```python
from build123d import *

# Parameters (mm, degrees)
SKETCH_W     = 65
SKETCH_H     = 56
SKETCH_R     = 1.5
PAD_DEPTH    = 1
FILLET_R     = 5
SKETCH001_W  = 40
SKETCH001_H  = 5
PAD001_DEPTH = 18
SKETCH002_W  = 5
SKETCH002_H  = 35
PAD002_DEPTH = 12


with BuildPart() as part:
    # Sketch → Pad (new body)
    with BuildSketch(Plane.XY):
        Rectangle(SKETCH_W, SKETCH_H)
        with Locations((-26.696429, 23)):
            Circle(SKETCH_R, mode=Mode.SUBTRACT)
        with Locations((-26.696429, -23)):
            Circle(SKETCH_R, mode=Mode.SUBTRACT)
        with Locations((26.696429, -23)):
            Circle(SKETCH_R, mode=Mode.SUBTRACT)
        with Locations((26.696429, 23)):
            Circle(SKETCH_R, mode=Mode.SUBTRACT)
    extrude(amount=PAD_DEPTH)

    # Fillet
    fillet_edges = [part.edges().sort_by_distance(p)[0] for p in [
        (-32.5, -28, 0.5),
        (32.5, -28, 0.5),
        (32.5, 28, 0.5),
        (-32.5, 28, 0.5),
    ]]
    fillet(fillet_edges, radius=FILLET_R)

    # Sketch001 (on Face5 of Fillet) → Pad001 (join)
    with BuildSketch(Plane.XY.offset(1)):
        with Locations((0, -23)):
            Rectangle(SKETCH001_W, SKETCH001_H)
    extrude(amount=PAD001_DEPTH)

    # Sketch002 (on Face2 of Pad001) → Pad002 (join)
    with BuildSketch(Plane(origin=(0, 0, 0), x_dir=(1, 0, 0), z_dir=(0, 0, -1))):
        with Locations((20, 0)):
            Rectangle(SKETCH002_W, SKETCH002_H)
    extrude(amount=PAD002_DEPTH)


solid = part.part
```
Geometry: final body of the model. Coordinates: model frame, mm. A direction names the side the tool comes from. Coordinates: 2 decimals unless noted, no trailing zeros. Order: outer loops, then holes, each group sorted by start corner. A loop starts at its lowest first (then second) coordinate and runs counter-clockwise, first axis right, second up. Notation, with made-up numbers: (68, 77.25) -> (109, 77.25) arc R24 cw to (109, 98.25) -> close; hole circle Ø2 at (38.5, -33). An arc over 180 degrees is marked (long way). Write each question's results on one line, items separated by ' | '. Start each with the question number.
1) Cut plane A-A, the plane y = -11.5. Output: boundary loops of the cut face in (x, z), and give its area (3 significant figures).
2) Mould query, pull axis X, two halves, no side actions, for faces 1 (the flat face through (-20, -23, 10)), 2 (the flat face through (0, -25.5, 10)), 3 (the cylindrical face through (27.503, 24.265, 0.493)). Classes: released by +X, released by -X, zero draft, split by the parting line, or undercut.
3) First-contact query: pin 1 (4 mm diameter, centred on x = 15, y = 10, fed in from -Z); pin 2 (4 mm diameter, centred on x = 19.5, z = -3.5, fed in from -Y); pin 3 (2.5 mm diameter, centred on y = -22.5, z = 13, fed in from +X). Flat tips, straight axial feed; report the tip coordinate or a pass-through.
4) Cut plane D-D, the plane z = 3. Output: boundary loops of the cut face in (x, y), and give its area (3 significant figures).
5) Cut plane C-C, the plane z = -3. Output: boundary loops of the cut face in (x, y).
6) Set-up query: faces 4 (the flat face through (17.5, 0, -6)), 5 (the flat face through (20, -17.5, -6)), 6 (the flat face through (0, -20.5, 10)), 7 (the flat face through (20, -23, 10)), 8 (the flat face through (20, 17.5, -6)). Return all of +Z, -Z, +X, -X, +Y, -Y with unobstructed straight access to the full face (end or side cutting, diameter ignored); none if empty.
7) Material intervals for line 1 along Y through (x, z) = (-15, 4); line 2 along X through (y, z) = (-14, -11); line 3 along Z through (x, y) = (-18, 22), sorted ascending.
8) Cut plane B-B, the plane x = 3.5. Output: boundary loops of the cut face in (y, z).
Checks:
1) outline: (-32.5, 0) -> (17.5, 0) -> (17.5, -12) -> (22.5, -12) -> (22.5, 0) -> (32.5, 0) -> (32.5, 1) -> (-32.5, 1) -> close | area: 125 mm^2
2) face 1: released by -X | face 2: zero draft | face 3: undercut
3) pin 1: z = 0 | pin 2: y = -17.5 | pin 3: x = 20
4) outline: (-20, -25.5) -> (20, -25.5) -> (20, -20.5) -> (-20, -20.5) -> close | area: 200 mm^2
5) outline: (17.5, -17.5) -> (22.5, -17.5) -> (22.5, 17.5) -> (17.5, 17.5) -> close
6) face 4: -Z, -X, +Y, -Y | face 5: -Z, +X, -X, -Y | face 6: +Z, +X, -X, +Y | face 7: +Z, +X, +Y, -Y | face 8: -Z, +X, -X, +Y
7) line 1: -25.5 to -20.5 | line 2: 17.5 to 22.5 | line 3: 0 to 1
8) outline: (-28, 0) -> (28, 0) -> (28, 1) -> (-20.5, 1) -> (-20.5, 19) -> (-25.5, 19) -> (-25.5, 1) -> (-28, 1) -> close
